Autodesk Inventor part; units mm, degrees
ref_plane "YZ Plane" through (0, 0, 0) normal (1, 0, 0) x (0, 1, 0)
ref_plane "XZ Plane" through (0, 0, 0) normal (0, 1, 0) x (-1, 0, 0)
ref_plane "XY Plane" through (0, 0, 0) normal (0, 0, 1) x (1, 0, 0)
sketch "Náčrt1" plane through (0, 0, 0) normal (0, 1, 0) x (-1, 0, 0)
  line L0 (0, 2.95) -> (-2.95, 2.95)
  line L1 (-2.95, 2.95) -> (-2.95, 0)
  line L2 (-2.95, 0) -> (0, 0)
  line L3 (0, 0) -> (0, 2.95)
  dimension "d0" = 2.95
  dimension "d1" = 2.95
extrude "Vysunutí1" add sketch "Náčrt1" along normal blind 6
sketch "Náčrt2" plane through (0, 6, 0) normal (0, 1, 0) x (1, 0, 0)
  line L0 (-1, -3.95) -> (3.95, -3.95)
  line L1 (3.95, -3.95) -> (3.95, 1)
  line L2 (3.95, 1) -> (-1, 1)
  line L3 (-1, 1) -> (-1, -3.95)
  line L4 (0, 0) -> (0, -2.95)
  line L5 (0, -2.95) -> (2.95, -2.95)
  line L6 (2.95, -2.95) -> (2.95, 0)
  line L7 (2.95, 0) -> (0, 0)
  dimension "d4" = 1
  dimension "d5" = 1
  dimension "d6" = 1
  dimension "d7" = 1
extrude "Vysunutí2" add sketch "Náčrt2" along normal blind 10 contours L3 L2 L1 L0 | L7 L6 L5 L4
sketch "Náčrt3" plane through (0, 16, 0) normal (0, 1, 0) x (1, 0, 0)
  line L0 (-4.05, 10.525) -> (17.95, 10.525)
  line L1 (17.95, 10.525) -> (17.95, -11.475)
  line L2 (17.95, -11.475) -> (-4.05, -11.475)
  line L3 (-4.05, -11.475) -> (-4.05, 10.525)
  line L4 (3.95, -3.95) -> (3.95, 1)
  line L5 (-1, -3.95) -> (3.95, -3.95)
  line L6 (3.95, 1) -> (-1, 1)
  line L7 (-1, 1) -> (-1, -3.95)
  point P0 (0, 0)
  dimension "d10" = 14
  dimension "d11" = 22
  dimension "d12" = 22
  dimension "d13" = 9.525
  dimension "d14" = 7.525
  dimension "d17" = 3.05
extrude "Vysunutí3" add sketch "Náčrt3" along normal blind 1 contours L0 L1 L2 L3 | L5 L7 L6 L4
equation "\"d1\" = d0"
equation "\"d5\" = d4"
equation "\"d6\" = d4"
equation "\"d7\" = d4"
equation "\"d12\" = d11"
properties part number "QRholderSpecial-top"
The model under review builds one solid part; all positions refer to its coordinate system, in mm. A direction names the side the tool comes from. Round coordinates to 2 decimals unless told otherwise and drop trailing zeros. Write each loop counter-clockwise with the first axis right and the second up, starting at its lowest first coordinate (ties: lowest second). Pieces come first, ordered by that corner, then holes.
(1) We need section C-C on y = 12.75. Give the boundary of the cut face in (x, z), and give its area (3 significant figures).
(2) Insertion check: pin 1 (2.5 mm diameter, centred on x = 1, y = 2, fed in from +Z); pin 2 (11 mm diameter, centred on x = 6.5, z = -4.5, fed in from -Y); pin 3 (2.5 mm diameter, centred on x = 2, y = 3, fed in from -Z). Each pin has a flat end and moves straight along its axis. Give the tip position at first contact, or say it passes through.
(3) We need section A-A on x = -0.5. Give the boundary of the cut face in (y, z) (3 decimals).
(4) We need section D-D on z = 0.75. Give the boundary of the cut face in (x, y), and give its area (3 significant figures).
(5) Wall thickness on L1, parallel to Z at x = 1.5, y = 1.5; L2, parallel to Y at x = -0.5, z = 3.25; L3, parallel to Y at x = -2.25, z = -8: over which ranges is each line inside the solid? List them lowest first.
(6) We need section B-B on z = 3.5. Give the boundary of the cut face in (x, y), and give its area (3 significant figures).
(7) Machinability: for faces 1 (the flat face through (-4.05, 16.5, 0.6)), 2 (the flat face through (1, 11, 3.95)), 3 (the flat face through (2.95, 3, 1)), 4 (the flat face through (1, 3, 0)), 5 (the flat face through (0, 3, 1)), which of the approach directions +Z, -Z, +X, -X, +Y, -Y give a long, thin tool a straight path to every point of the face, cutting with its end or side? Answer none if there is none.
Findings below:
1. outline: (-1, -1) - (3.95, -1) - (3.95, 3.95) - (-1, 3.95) - close
1. area: 24.5 mm2
2. pin 1: stops at z = 2.95
2. pin 2: stops at y = 6
2. pin 3: stops at z = 0
3. outline: (6, -1) - (16, -1) - (16, -10.525) - (17, -10.525) - (17, 11.475) - (16, 11.475) - (16, 3.95) - (6, 3.95) - close
4. outline: (-4.05, 16) - (-1, 16) - (-1, 6) - (0, 6) - (0, 0) - (2.95, 0) - (2.95, 6) - (3.95, 6) - (3.95, 16) - (17.95, 16) - (17.95, 17) - (-4.05, 17) - close
4. area: 89.2 mm2
5. L1: z = 0 to 2.95
5. L2: y = 6 to 17
5. L3: y = 16 to 17
6. outline: (-4.05, 16) - (-1, 16) - (-1, 6) - (3.95, 6) - (3.95, 16) - (17.95, 16) - (17.95, 17) - (-4.05, 17) - close
6. area: 71.5 mm2
7. face 1: +Z, -Z, -X, +Y, -Y
7. face 2: +Z, +X, -X, -Y
7. face 3: +Z, -Z, +X, -Y
7. face 4: -Z, +X, -X, -Y
7. face 5: +Z, -Z, -X, -Y
